from build123d import *

# Parameters (mm, degrees)
F0_W          = 67.630976
F0_H          = 58.502942
F1_DEPTH      = 101.344071
F1_DEPTH_BACK = 102.304079
F2_R          = 21.597403
F3_DEPTH      = 6.715551


with BuildPart() as f1:
    # F0 (on Top) → F1 (new body, two sides)
    with BuildSketch(Plane.XY) as f1_sk:
        Rectangle(F0_W, F0_H)
    extrude(amount=F1_DEPTH)
    extrude(f1_sk.sketch, amount=-F1_DEPTH_BACK)

    # F2 (on face) → F3 (join)
    with BuildSketch(Plane.YZ.offset(33.815488)):
        with Locations((0, 68.826675)):
            Circle(F2_R)
        with Locations((0, -68.826675)):
            Circle(F2_R)
    extrude(amount=F3_DEPTH)


solid = f1.part
Work out the finished part from the listing and answer in its coordinate system (mm). A direction names the side the tool comes from. Round coordinates to 2 decimals unless told otherwise and drop trailing zeros. Order: outer loops, then holes, each group sorted by start corner. A loop starts at its lowest first (then second) coordinate and runs counter-clockwise, first axis right, second up. Notation, with made-up numbers: M -18,-38.5 L -14,-38.5 A17 ccw -14,-33.5 Z; hole C -18.75,-33 d5. An arc over 180 degrees is marked long. One line per item, written item: value.
Q1. Find section C-C on z = -31. Write down the section's boundary in (x, y), then the cut area to 3 significant figures.
Derived:
outline: M -33.82,-29.25 L 33.82,-29.25 L 33.82,29.25 L -33.82,29.25 Z
area: 3,960 mm²
Q2. Find section B-B on z = 86. Write down the section's boundary in (x, y), then the cut area to 3 significant figures.
Derived:
outline: M -33.82,-29.25 L 33.82,-29.25 L 33.82,-13.1 L 40.53,-13.1 L 40.53,13.1 L 33.82,13.1 L 33.82,29.25 L -33.82,29.25 Z
area: 4,130 mm²
Q3. For faces 4 (the face through (40.531, 0, 69)), 5 (the face through (37.13, -4.68, -89.91)), determine the directions among +Z, -Z, +X, -X, +Y, -Y from which every point of the face is accessible in a straight line to the end or side of a thin tool.
Derived:
face 4: +Z, -Z, +X, +Y, -Y
face 5: +X
Q4. Straight lines are drawn through the part: line 1 (X direction, y = 23.5, z = 3); line 2 (Y direction, x = 36.5, z = 68); line 3 (Z direction, x = 35, y = 10.5). For each, find the intervals that lie inside material, in ascending order.
Derived:
line 1: -33.82 to 33.82
line 2: -21.58 to 21.58
line 3: -87.7 to -49.95, 49.95 to 87.7
Q5. Find section D-D on z = -59. Write down the section's boundary in (x, y).
Derived:
outline: M -33.82,-29.25 L 33.82,-29.25 L 33.82,-19.23 L 40.53,-19.23 L 40.53,19.23 L 33.82,19.23 L 33.82,29.25 L -33.82,29.25 Z
Q6. Determine the mould class of faces 1 (the face through (-33.815, 0, 1)), 2 (the face through (0, 0, 101.344)), 3 (the face through (33.815, 0, 1)) for opening direction Z: released by +Z, released by -Z, zero draft, split by the parting line, or undercut.
Derived:
face 1: zero draft
face 2: released by +Z
face 3: undercut
Q7. Find section A-A on y = 0. Write down the section's boundary in (x, z), then the cut area to 3 significant figures.
Derived:
outline: M -33.82,-102.3 L 33.82,-102.3 L 33.82,-90.42 L 40.53,-90.42 L 40.53,-47.23 L 33.82,-47.23 L 33.82,47.23 L 40.53,47.23 L 40.53,90.42 L 33.82,90.42 L 33.82,101.34 L -33.82,101.34 Z
area: 14,400 mm²
